Autodesk Inventor part; units mm, degrees
ref_plane "YZ Plane" through (0, 0, 0) normal (1, 0, 0) x (0, 1, 0)
ref_plane "XZ Plane" through (0, 0, 0) normal (0, 1, 0) x (-1, 0, 0)
ref_plane "XY Plane" through (0, 0, 0) normal (0, 0, 1) x (1, 0, 0)
sketch "Sketch2" plane through (0, 0, 0) normal (0, 0, 1) x (1, 0, 0)
  line L0 (-105, -72.5) -> (105, -72.5)
  line L1 (105, -72.5) -> (105, 72.5)
  line L2 (105, 72.5) -> (-105, 72.5)
  line L3 (-105, 72.5) -> (-105, -72.5)
  line L4 (-105, -72.5) -> (105, 72.5) construction
  line L5 (105, -72.5) -> (-105, 72.5) construction
  point P0 (0, 0)
  dimension "d11" = 145
  dimension "d12" = 210
extrude "Extrusion2" add sketch "Sketch2" along normal blind 8
sketch "Sketch3" plane through (0, 0, 8) normal (0, 0, 1) x (1, 0, 0)
  line L0 (105, 72.5) -> (-105, 72.5)
  line L1 (-63, 72.5) -> (-21, 72.5)
  line L2 (-21, 72.5) -> (-21, 80.5)
  line L3 (-21, 80.5) -> (-63, 80.5)
  line L4 (-63, 80.5) -> (-63, 72.5)
  line L5 (63, 72.5) -> (21, 72.5)
  line L6 (21, 72.5) -> (21, 80.5)
  line L7 (21, 80.5) -> (63, 80.5)
  line L8 (63, 80.5) -> (63, 72.5)
  line L9 (-21, 80.5) -> (21, 80.5) construction
  line L10 (63, 80.5) -> (105, 80.5) construction
  line L11 (-63, 80.5) -> (-105, 80.5) construction
  point P0 (0, 0)
  dimension "d15" = 8
extrude "Extrusion3" add sketch "Sketch3" against normal blind 8
mirror "Mirror1" about plane through (0, 0, 0) normal (0, 1, 0) of "Extrusion3"
sketch "Sketch4" plane through (0, 0, 8) normal (0, 0, 1) x (1, 0, 0)
  line L0 (-105, 72.5) -> (-105, -72.5)
  line L1 (-105, 24.1667) -> (-97, 24.1667)
  line L2 (-97, 24.1667) -> (-97, -24.1667)
  line L3 (-97, -24.1667) -> (-105, -24.1667)
  line L4 (-105, -24.1667) -> (-105, 24.1667)
  line L5 (-97, 24.1667) -> (-97, 72.5) construction
  line L6 (-97, -24.1667) -> (-97, -72.5) construction
  point P0 (0, 0)
  dimension "d20" = 8
extrude "Extrusion4" cut sketch "Sketch4" against normal blind 8
mirror "Mirror2" about plane through (0, 0, 0) normal (1, 0, 0) of "Extrusion4"
properties part number "M06 - Wall Side 1" material "Wood (Walnut)"
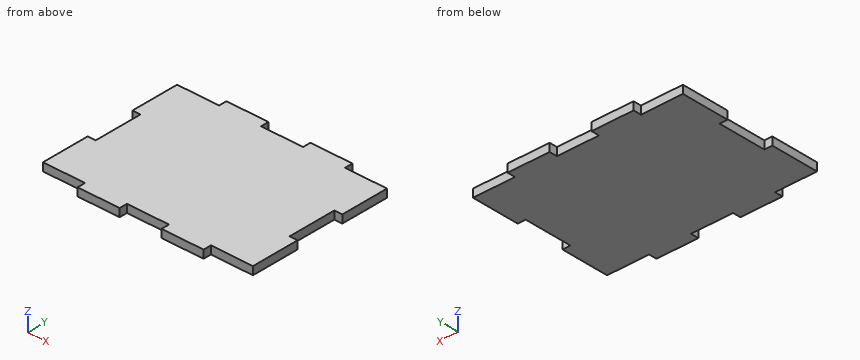
Read the model definition and answer for the solid it produces. Units are mm, in the model's axes. Give positions to 0.01 mm unless a question says otherwise; leave off trailing zeros. Write each loop counter-clockwise with the first axis right and the second up, starting at its lowest first coordinate (ties: lowest second). Pieces come first, ordered by that corner, then holes. Notation, with made-up numbers: M -2,-18.75 L 29,-18.75 A13 ccw 29,-7.75 Z; hole C 84.25,-17 d2. An arc over 180 degrees is marked long. Put each result on its own line as item: value. Start each with the question number.
1. Each of these flat-tipped pins is pushed along its axis until it touches: pin 1 Ø4 at (x, z) = (100, 5) entering from +Y; pin 2 Ø4 at (y, z) = (-78.5, 2) entering from +X; pin 3 Ø4 at (y, z) = (8.5, 6) entering from -X. Where does it stop, or does it pass through?
2. The part is cut by section C-C, the plane y = -2. Give the vertices of the cut face in (x, z).
3. The part is cut by section A-A, the plane z = 5.5. Give the vertices of the cut face in (x, y), and give its area (3 significant figures).
4. Consider line 1 along Y through (x, z) = (-87, 4.5); line 2 along X through (y, z) = (-11.5, 6.75). Determine where each line is inside the solid, lowest interval first.
5. The part is cut by section B-B, the plane x = -1.5. Give the vertices of the cut face in (y, z).
Final values:
1. pin 1: stops at y = 72.5
1. pin 2: stops at x = 63
1. pin 3: stops at x = -97
2. outline: M -97,0 L 97,0 L 97,8 L -97,8 Z
3. outline: M -105,-72.5 L -63,-72.5 L -63,-80.5 L -21,-80.5 L -21,-72.5 L 21,-72.5 L 21,-80.5 L 63,-80.5 L 63,-72.5 L 105,-72.5 L 105,-24.17 L 97,-24.17 L 97,24.17 L 105,24.17 L 105,72.5 L 63,72.5 L 63,80.5 L 21,80.5 L 21,72.5 L -21,72.5 L -21,80.5 L -63,80.5 L -63,72.5 L -105,72.5 L -105,24.17 L -97,24.17 L -97,-24.17 L -105,-24.17 Z
3. area: 31,000 mm²
4. line 1: y = -72.5 to 72.5
4. line 2: x = -97 to 97
5. outline: M -72.5,0 L 72.5,0 L 72.5,8 L -72.5,8 Z
